Verification items for the finished model (mm, model axes). A direction names the side the tool comes from. Give positions to 0.01 mm unless a question says otherwise; leave off trailing zeros. Order: outer loops, then holes, each group sorted by start corner. A loop starts at its lowest first (then second) coordinate and runs counter-clockwise, first axis right, second up.
from build123d import *

# Parameters (mm, degrees)
F1_DEPTH = 10
F2_R     = 5
F3_R     = 2
F4_R     = 10
F5_R     = 1
F6_R     = 10


with BuildPart() as f1:
    # F0 (on Front) → F1 (new body)
    with BuildSketch(Plane.XZ):
        Polygon((-27.5, 34.135083), (-27.5, -29.821047), (34.5, -29.821047), (34.5, -1.869009), (20.437485, 2.430633), (34.5, 8.652056), (34.5, 34.135083), align=None)
        Polygon((-20.5, 27.135083), (27.5, 27.135083), (27.5, 12.135083), (11, 12.135083), (11, 5.930633), (17.350806, 5.930633), (17.350806, -1.069367), (11, -1.069367), (11, -7.821047), (27.5, -7.821047), (27.5, -22.821047), (-20.5, -22.821047), align=None, mode=Mode.SUBTRACT)
    extrude(amount=F1_DEPTH)

    # F2
    f2_edges = [f1.edges().sort_by_distance(p)[0] for p in [
        (-20.5, -5, 27.135083),
        (27.5, -5, 27.135083),
        (27.5, -5, 12.135083),
        (-20.5, -5, -22.821047),
        (27.5, -5, -22.821047),
        (27.5, -5, -7.821047),
    ]]
    fillet(f2_edges, radius=F2_R)

    # F3
    f3_edges = [f1.edges().sort_by_distance(p)[0] for p in [
        (11, -5, 12.135083),
        (11, -5, 5.930633),
        (17.350806, -5, 5.930633),
        (17.350806, -5, -1.069367),
        (11, -5, -1.069367),
        (11, -5, -7.821047),
    ]]
    fillet(f3_edges, radius=F3_R)

    # F4
    f4_edges = [f1.edges().sort_by_distance(p)[0] for p in [
        (34.5, -5, 34.135083),
        (34.5, -5, 8.652056),
        (34.5, -5, -1.869009),
        (34.5, -5, -29.821047),
    ]]
    fillet(f4_edges, radius=F4_R)

    # F5
    f5_edges = [f1.edges().sort_by_distance(p)[0] for p in [
        (20.437485, -5, 2.430633),
    ]]
    fillet(f5_edges, radius=F5_R)

    # F6
    f6_edges = [f1.edges().sort_by_distance(p)[0] for p in [
        (-27.5, -5, 34.135083),
        (-27.5, -5, -29.821047),
    ]]
    fillet(f6_edges, radius=F6_R)


solid = f1.part
(1) Go/stop test with flat-tipped pins: pin 1 (3 mm diameter, centred on y = -5, z = 9, fed in from +X); pin 2 (6 mm diameter, centred on y = -2.5, z = 12, fed in from +X). Record where each tip stops, or that it passes through.
Solved:
pin 1: stops at x = 33.35
pin 2: stops at x = 34.5
(2) Set-up check for faces 1 (the flat face through (27.5, -5, -15)), 2 (the flat face through (25.68, -4.93, 4.75)), 3 (the flat face through (17, -10, 10)): record each of +Z, -Z, +X, -X, +Y, -Y from which the full face is reachable in a straight line by a thin tool's end or side.
Solved:
face 1: +Y, -Y
face 2: +X, +Y, -Y
face 3: +Z, -Z, +X, -X, -Y
(3) Release check for a two-part mould opening along X. For faces 4 (the flat face through (17.351, -5, 2)), 5 (the cylindrical face through (22.298, -5.07, 2.559)), 6 (the cylindrical face through (-24.493, -5.07, 31.283)) record: pulls with the +X half, pulls with the -X half, needs draft (parallel to the pull), parting line crosses it, or undercut.
Solved:
face 4: undercut
face 5: pulls with the +X half
face 6: pulls with the -X half
(4) Section check B-B, the plane x = -22. Enter the section's corners in (y, z), then the cut area to 3 significant figures.
Solved:
outline: (-10, -28.75) - (0, -28.75) - (0, 33.07) - (-10, 33.07) - close
area: 618 mm2
(5) Scan lines: line 1 (Z direction, x = 13, y = -9.25); line 2 (Z direction, x = -9, y = -6); line 3 (X direction, y = -2.75, z = -13.5). Record each from-to range of solid material in increasing order.
Solved:
line 1: z = -29.82 to -22.82, -7.82 to -1.07, 5.93 to 12.14, 27.14 to 34.14
line 2: z = -29.82 to -22.82, 27.14 to 34.14
line 3: x = -27.5 to -20.5, 27.5 to 34.5
(6) Section check A-A, the plane x = -13. Enter the section's corners in (y, z).
Solved:
outline: (-10, -29.82) - (0, -29.82) - (0, -22.82) - (-10, -22.82) - close; (-10, 27.14) - (0, 27.14) - (0, 34.14) - (-10, 34.14) - close
